Part model, mm, in its own coordinate system. A direction names the side the tool comes from. Coordinates: 2 decimals unless noted, no trailing zeros. Write each loop counter-clockwise with the first axis right and the second up, starting at its lowest first coordinate (ties: lowest second). Pieces come first, ordered by that corner, then holes. Notation, with made-up numbers: (-10.5, 57) - (34.5, 57) arc R20 cw to (34.5, 81) - close; hole circle Ø1 at (54.25, 22.25). An arc over 180 degrees is marked (long way). Use a Markdown table: item, result.
```python
from build123d import *

# Parameters (mm, degrees)
EXTRUDE_1_DEPTH     = 13
SKETCH_2_R          = 2.525
CUT_EXTRUDE_1_DEPTH = 14
CUT_EXTRUDE_2_DEPTH = 14
SKETCH_4_R          = 2.525
CUT_EXTRUDE_3_DEPTH = 14
SKETCH_5_W          = 8
SKETCH_5_H          = 50
CUT_EXTRUDE_4_DEPTH = 14
SKETCH_6_R          = 1.525
CUT_EXTRUDE_5_DEPTH = 14
SKETCH_7_W          = 12
SKETCH_7_H          = 55
CUT_EXTRUDE_6_DEPTH = 14
FILLET_1_R          = 20
FILLET_2_R          = 20
FILLET_3_R          = 2


with BuildPart() as part:
    # 草图1 → 凸台-拉伸1 (new body)
    with BuildSketch(Plane(origin=(0, 0, 0), x_dir=(1, 0, 0), z_dir=(0, 1, 0))):
        with BuildLine():
            ThreePointArc((16.583123952, 25), (-30, 0), (16.583123952, -25))
            Line((16.583123952, -25), (16.583123952, 25))
        make_face()
        with BuildLine():
            Line((16.583123952, 25), (16.583123952, -25))
            ThreePointArc((16.583123952, -25), (26.433820369, -14.186371655), (30, 0))
            ThreePointArc((30, 0), (26.433820369, 14.186371655), (16.583123952, 25))
        make_face()
        with BuildLine():
            ThreePointArc((30, 0), (26.433820369, -14.186371655), (16.583123952, -25))
            Line((16.583123952, -25), (70, -25))
            Line((70, -25), (70, 25))
            Line((70, 25), (16.583123952, 25))
            ThreePointArc((16.583123952, 25), (26.433820369, 14.186371655), (30, 0))
        make_face()
    extrude(amount=EXTRUDE_1_DEPTH)

    # 草图2 → 切除-拉伸1 (cut, through all)
    with BuildSketch(Plane(origin=(0, 13, 0), x_dir=(1, 0, 0), z_dir=(0, 1, 0))):
        with Locations((-25.75, 0)):
            Circle(SKETCH_2_R)
        with Locations((-12.875, 22.300154147)):
            Circle(SKETCH_2_R)
        with Locations((12.875, 22.300154147)):
            Circle(SKETCH_2_R)
        with Locations((25.75, 0)):
            Circle(SKETCH_2_R)
        with Locations((12.875, -22.300154147)):
            Circle(SKETCH_2_R)
        with Locations((-12.875, -22.300154147)):
            Circle(SKETCH_2_R)
    extrude(amount=-CUT_EXTRUDE_1_DEPTH, mode=Mode.SUBTRACT)

    # 草图3 → 切除-拉伸2 (cut, through all)
    with BuildSketch(Plane(origin=(0, 13, 0), x_dir=(1, 0, 0), z_dir=(0, 1, 0))):
        with BuildLine():
            Line((13.784048752, -16.5), (52, -16.5))
            Line((52, -16.5), (52, 16.5))
            Line((52, 16.5), (13.784048752, 16.5))
            ThreePointArc((13.784048752, 16.5), (-21.5, 0), (13.784048752, -16.5))
        make_face()
    extrude(amount=-CUT_EXTRUDE_2_DEPTH, mode=Mode.SUBTRACT)

    # 草图4 → 切除-拉伸3 (cut, through all)
    with BuildSketch(Plane(origin=(0, 13, 0), x_dir=(1, 0, 0), z_dir=(0, 1, 0))):
        with Locations((45.5, 21.1)):
            Circle(SKETCH_4_R)
        with Locations((45.5, -21.1)):
            Circle(SKETCH_4_R)
    extrude(amount=-CUT_EXTRUDE_3_DEPTH, mode=Mode.SUBTRACT)

    # 草图5 → 切除-拉伸4 (cut, through all)
    with BuildSketch(Plane(origin=(0, 13, 0), x_dir=(1, 0, 0), z_dir=(0, 1, 0))):
        with Locations((66, 0)):
            Rectangle(SKETCH_5_W, SKETCH_5_H)
    extrude(amount=-CUT_EXTRUDE_4_DEPTH, mode=Mode.SUBTRACT)

    # 草图6 → 切除-拉伸5 (cut, through all)
    with BuildSketch(Plane(origin=(0, 13, 0), x_dir=(1, 0, 0), z_dir=(0, 1, 0))):
        with Locations((56, 0)):
            Circle(SKETCH_6_R)
        with Locations((56, 15)):
            Circle(SKETCH_6_R)
        with Locations((56, -15)):
            Circle(SKETCH_6_R)
    extrude(amount=-CUT_EXTRUDE_5_DEPTH, mode=Mode.SUBTRACT)

    # 草图7 → 切除-拉伸6 (cut, through all)
    with BuildSketch(Plane(origin=(0, 13, 0), x_dir=(1, 0, 0), z_dir=(0, 1, 0))):
        with Locations((56, -2.5)):
            Rectangle(SKETCH_7_W, SKETCH_7_H)
    extrude(amount=-CUT_EXTRUDE_6_DEPTH, mode=Mode.SUBTRACT)

    # 圆角1
    fillet_1_edges = [part.edges().sort_by_distance(p)[0] for p in [
        (13.784048752, 6.5, -16.5),
        (13.784048752, 6.5, 16.5),
    ]]
    fillet(fillet_1_edges, radius=FILLET_1_R)

    # 圆角2
    fillet_2_edges = [part.edges().sort_by_distance(p)[0] for p in [
        (16.583123952, 6.5, -25),
        (16.583123952, 6.5, 25),
    ]]
    fillet(fillet_2_edges, radius=FILLET_2_R)

    # 圆角3
    fillet_3_edges = [part.edges().sort_by_distance(p)[0] for p in [
        (50, 6.5, 16.5),
        (50, 6.5, 25),
        (50, 6.5, -16.5),
        (50, 6.5, -25),
    ]]
    fillet(fillet_3_edges, radius=FILLET_3_R)


solid = part.part
```
Item 1: Which spindle directions (+Z, -Z, +X, -X, +Y, -Y) get a long thin tool onto all of the face, cutting with end or side? Do faces 1 (the face through (17.384, 6.591, -25.492)), 2 (the face through (49.43, 6.59, 17.1)), 3 (the face through (14.907, 6.409, -17.095)), 4 (the face through (35, 6, 25)). Say none if no direction does.
From the geometry:
| item | result |
|---|---|
| face 1 | -Z, +X, +Y, -Y |
| face 2 | +X, +Y, -Y |
| face 3 | +Y, -Y |
| face 4 | +Z, +X, +Y, -Y |
Item 2: Drop flat-ended pins along their axis: P1, Ø1, axis at x = 11.5, y = 9, coming from the -Z side; P2, Ø4, axis at x = 18, y = 4.5, coming from the +Z side; P3, Ø6, axis at x = 45.5, z = -21.1, coming from the +Y side; P4, Ø5, axis at y = 8, z = -7.5, coming from the +X side. Give the stop position or say it passes through.
From the geometry:
| item | result |
|---|---|
| P1 | z = -27.91 |
| P2 | z = 25.86 |
| P3 | y = 13 |
| P4 | x = -19.03 |
Item 3: Band-saw the part on C-C, the plane x = 37. Give the cut face in (y, z), then the cut area to 3 significant figures.
From the geometry:
| item | result |
|---|---|
| outline | (0, -25) - (13, -25) - (13, -16.5) - (0, -16.5) - close; (0, 16.5) - (13, 16.5) - (13, 25) - (0, 25) - close |
| area | 221 mm^2 |
Item 4: Band-saw the part on A-A, the plane x = 45.5. Give the cut face in (y, z) (3 decimals).
From the geometry:
| item | result |
|---|---|
| outline | (0, -25) - (13, -25) - (13, -23.625) - (0, -23.625) - close; (0, -18.575) - (13, -18.575) - (13, -16.5) - (0, -16.5) - close; (0, 16.5) - (13, 16.5) - (13, 18.575) - (0, 18.575) - close; (0, 23.625) - (13, 23.625) - (13, 25) - (0, 25) - close |
Item 5: Drill centre lines: probe 1 along Z at (x, y) = (45.5, 6.75) (3 decimals); probe 2 along X at (y, z) = (9, 23); probe 3 along Z at (x, y) = (41, 5.25). Where is each one in solid material? Low to high.
From the geometry:
| item | result |
|---|---|
| probe 1 | -25 to -23.625, -18.575 to -16.5, 16.5 to 18.575, 23.625 to 25 |
| probe 2 | -19.26 to -15.3, -10.45 to 10.45, 15.3 to 43.84, 47.16 to 50 |
| probe 3 | -25 to -16.5, 16.5 to 25 |
Item 6: Band-saw the part on D-D, the plane y = 7.75. Count the separate pieces of the cut face and the enclosed holes in it, then the cut area to 3 significant figures.
From the geometry:
| item | result |
|---|---|
| separate pieces | 1 |
| enclosed holes | 7 |
| area | 1,410 mm^2 |
Item 7: Two-plate mould, pull along X, no slides. Class faces 5 (the face through (35, 6, -25)), 6 (the face through (-15.4, 6.6, -22.4)), 7 (the face through (17.26, 6.59, 25.52)): pulls with the +X half, pulls with the -X half, needs draft (parallel to the pull), parting line crosses it, or undercut.
From the geometry:
| item | result |
|---|---|
| face 5 | needs draft |
| face 6 | undercut |
| face 7 | pulls with the +X half |
Item 8: Band-saw the part on B-B, the plane z = 0. Give the cut face in (x, y) (3 decimals), then the cut area to 4 significant figures.
From the geometry:
| item | result |
|---|---|
| outline | (-30, 0) - (-28.275, 0) - (-28.275, 13) - (-30, 13) - close; (-23.225, 0) - (-21.5, 0) - (-21.5, 13) - (-23.225, 13) - close |
| area | 44.85 mm^2 |
